```python
from build123d import *

# Parameters (mm, degrees)
EXTRUDE_1_DEPTH          = 5
SKETCH_2_R               = 7
EXTRUDE_2_DEPTH          = 30
EXTRUDE_3_DEPTH          = 5
EXTRUDE_4_DEPTH          = 55
SKETCH_5_R               = 2
CUT_EXTRUDE_1_DEPTH      = 169.861141178
EXTRUDE_5_DEPTH          = 40
CUT_EXTRUDE_2_DEPTH      = 161.374826578
CUT_EXTRUDE_2_DEPTH_BACK = 161.374826578


with BuildPart() as part:
    # Эскиз1 → Бобышка-Вытянуть1 (new body)
    with BuildSketch(Plane.XY):
        with BuildLine():
            Line((-118.25, -20), (118.25, -20))
            ThreePointArc((118.25, -20), (138.25, 0), (118.25, 20))
            Line((118.25, 20), (-118.25, 20))
            ThreePointArc((-118.25, 20), (-138.25, 0), (-118.25, -20))
        make_face()
    extrude(amount=EXTRUDE_1_DEPTH)

    # Эскиз2 → Бобышка-Вытянуть2 (add)
    with BuildSketch(Plane(origin=(0, 0, 0), x_dir=(-1, 0, 0), z_dir=(0, 0, -1))):
        with Locations(Location((-118.25, 0, 0), (0, 0, 180))):
            Circle(SKETCH_2_R)
        with Locations(Location((118.25, 0, 0), (0, 0, 180))):
            Circle(SKETCH_2_R)
    extrude(amount=EXTRUDE_2_DEPTH)

    # Эскиз3 → Бобышка-Вытянуть3 (add)
    with BuildSketch(Plane.XY.offset(5)):
        Polygon((-118.25, 20), (-78.4, 59.85), (78.4, 59.85), (118.25, 20), align=None)
    extrude(amount=-EXTRUDE_3_DEPTH)

    # Эскиз4 → Бобышка-Вытянуть4 (add)
    with BuildSketch(Plane(origin=(0, 0, 0), x_dir=(-1, 0, 0), z_dir=(0, 0, -1))):
        Polygon((-78.4, 59.85), (-83.4, 54.85), (83.4, 54.85), (78.4, 59.85), align=None)
    extrude(amount=EXTRUDE_4_DEPTH)

    # Эскиз5 → Вырез-Вытянуть1 (cut, through all)
    with BuildSketch(Plane(origin=(0, 59.85, 0), x_dir=(1, 0, 0), z_dir=(0, 1, 0))):
        with Locations(Location((0, 50, 0), (0, 0, 180))):
            Circle(SKETCH_5_R)
        with Locations(Location((8, 50, 0), (0, 0, 180))):
            Circle(SKETCH_5_R)
        with Locations(Location((16, 50, 0), (0, 0, 180))):
            Circle(SKETCH_5_R)
        with Locations(Location((24, 50, 0), (0, 0, 180))):
            Circle(SKETCH_5_R)
        with Locations(Location((32, 50, 0), (0, 0, 180))):
            Circle(SKETCH_5_R)
        with Locations(Location((40, 50, 0), (0, 0, 180))):
            Circle(SKETCH_5_R)
        with Locations(Location((48, 50, 0), (0, 0, 180))):
            Circle(SKETCH_5_R)
        with Locations(Location((56, 50, 0), (0, 0, 180))):
            Circle(SKETCH_5_R)
        with Locations(Location((64, 50, 0), (0, 0, 180))):
            Circle(SKETCH_5_R)
        with Locations(Location((-8, 50, 0), (0, 0, 180))):
            Circle(SKETCH_5_R)
        with Locations(Location((-16, 50, 0), (0, 0, 180))):
            Circle(SKETCH_5_R)
        with Locations(Location((-24, 50, 0), (0, 0, 180))):
            Circle(SKETCH_5_R)
        with Locations(Location((-32, 50, 0), (0, 0, 180))):
            Circle(SKETCH_5_R)
        with Locations(Location((-40, 50, 0), (0, 0, 180))):
            Circle(SKETCH_5_R)
        with Locations(Location((-48, 50, 0), (0, 0, 180))):
            Circle(SKETCH_5_R)
        with Locations(Location((-56, 50, 0), (0, 0, 180))):
            Circle(SKETCH_5_R)
        with Locations(Location((-64, 50, 0), (0, 0, 180))):
            Circle(SKETCH_5_R)
    extrude(amount=-CUT_EXTRUDE_1_DEPTH, mode=Mode.SUBTRACT)

    # Эскиз7 → Бобышка-Вытянуть5 (add)
    with BuildSketch(Plane(origin=(0, 0, 0), x_dir=(-1, 0, 0), z_dir=(0, 0, -1))):
        Polygon((-118.25, 20), (-111.178932188, 20), (-76.04842613, 55.130506058), (-83.4, 54.85), align=None)
        Polygon((83.4, 54.85), (76.328932188, 54.85), (111.178932188, 20), (118.25, 20), align=None)
    extrude(amount=EXTRUDE_5_DEPTH)

    # Эскиз10 → Вырез-Вытянуть2 (cut, two sides: drawn at the far end of the back side and taken through both)
    with BuildSketch(Plane(origin=(0, 0, 0), x_dir=(0, 0, -1), z_dir=(1, 0, 0)).offset(-CUT_EXTRUDE_2_DEPTH_BACK)):
        Polygon((0, 20), (40, 20), (40, 54.85), (0, 45), align=None)
    extrude(amount=CUT_EXTRUDE_2_DEPTH + CUT_EXTRUDE_2_DEPTH_BACK, mode=Mode.SUBTRACT)


solid = part.part
```
Check sheet for the modelled part. Datum: model origin and axes. Units: mm. A direction names the side the tool comes from. Round coordinates to 2 decimals unless told otherwise and drop trailing zeros. Loops run counter-clockwise (first coordinate to the right, second up) from the corner with the lowest first, then second, coordinate; pieces in that order, holes last. Notation, with made-up numbers: (7, 67.5) - (26, 67.5) arc R20 cw to (26, 89.5) - close; hole circle Ø11 at (14, -14.5). An arc over 180 degrees is marked (long way). Answer as a JSON object with one key per item and string values. Group by question number.
Q1. Mould release check, pull along X, two halves, no side actions. Record for faces 1 (the face through (1, 57, -55)), 2 (the face through (86.42, 51.83, -13.75)), 3 (the face through (-88.09, 50.16, -15.97)), 4 (the face through (2, 18, 0)): released by +X, released by -X, zero draft, split by the parting line, or undercut.
Q2. Sectioned sample at A-A, the plane y = 0. Enter the section's corners in (x, z).
Q3. Scan lines: line 1 along Z through (x, y) = (-24, 56.45); line 2 along Z through (x, y) = (11.5, 19); line 3 along Y through (x, z) = (-23, -35.5). Record each from-to range of solid material in increasing order. Write a range as [from, to].
Q4. Sectioned sample at B-B, the plane z = -9.5. Enter the section's corners in (x, y), plus the area to 3 significant figures.
Q5. Gauge pin test, flat ends, axial feed: P1, Ø12, axis at y = -6, z = -21, coming from the -X side; P2, Ø10, axis at x = -2.5, y = 4.5, coming from the -Z side; P3, Ø12, axis at x = -94, z = -16.5, coming from the -Y side. Record the tip position at first contact, or that the pin passes through.
Q6. Set-up check for faces 5 (the face through (111.257, -0.308, -14.79)), 6 (the face through (79.134, 52.045, -10.831)), 7 (the face through (84.7, 50, -20.3)): record each of +Z, -Z, +X, -X, +Y, -Y from which the full face is reachable in a straight line by a thin tool's end or side.
Q7. Sectioned sample at C-C, the plane x = 81. Enter the section's corners in (y, z), plus the area to 3 significant figures.
Solution:
{
 "1": {"face 1": "zero draft", "face 2": "released by +X", "face 3": "released by -X", "face 4": "undercut"},
 "2": {"outline": "(-138.25, 0) - (-125.25, 0) - (-125.25, -30) - (-111.25, -30) - (-111.25, 0) - (111.25, 0) - (111.25, -30) - (125.25, -30) - (125.25, 0) - (138.25, 0) - (138.25, 5) - (-138.25, 5) - close"},
 "3": {"line 1": "z = [-55, -52], [-48, 5]", "line 2": "z = [0, 5]", "line 3": "y = [54.85, 59.85]"},
 "4": {"outline": "circle Ø14 at (-118.25, 0); (-90.91, 47.34) - (-83.84, 47.34) - (-76.33, 54.85) - (76.33, 54.85) - (83.84, 47.34) - (90.91, 47.34) - (78.4, 59.85) - (-78.4, 59.85) - close; circle Ø14 at (118.25, 0)", "area": "1,220 mm²"},
 "5": {"P1": "stops at x = -125.25", "P2": "stops at z = 0", "P3": "stops at y = 47.89"},
 "6": {"face 5": "-Z", "face 6": "-Z, -Y", "face 7": "-Z, +X, -X, -Y"},
 "7": {"outline": "(-20, 0) - (50.18, 0) - (50.18, -21.03) - (54.85, -40) - (54.85, -55) - (57.25, -55) - (57.25, 5) - (-20, 5) - close", "area": "661 mm²"}
}
